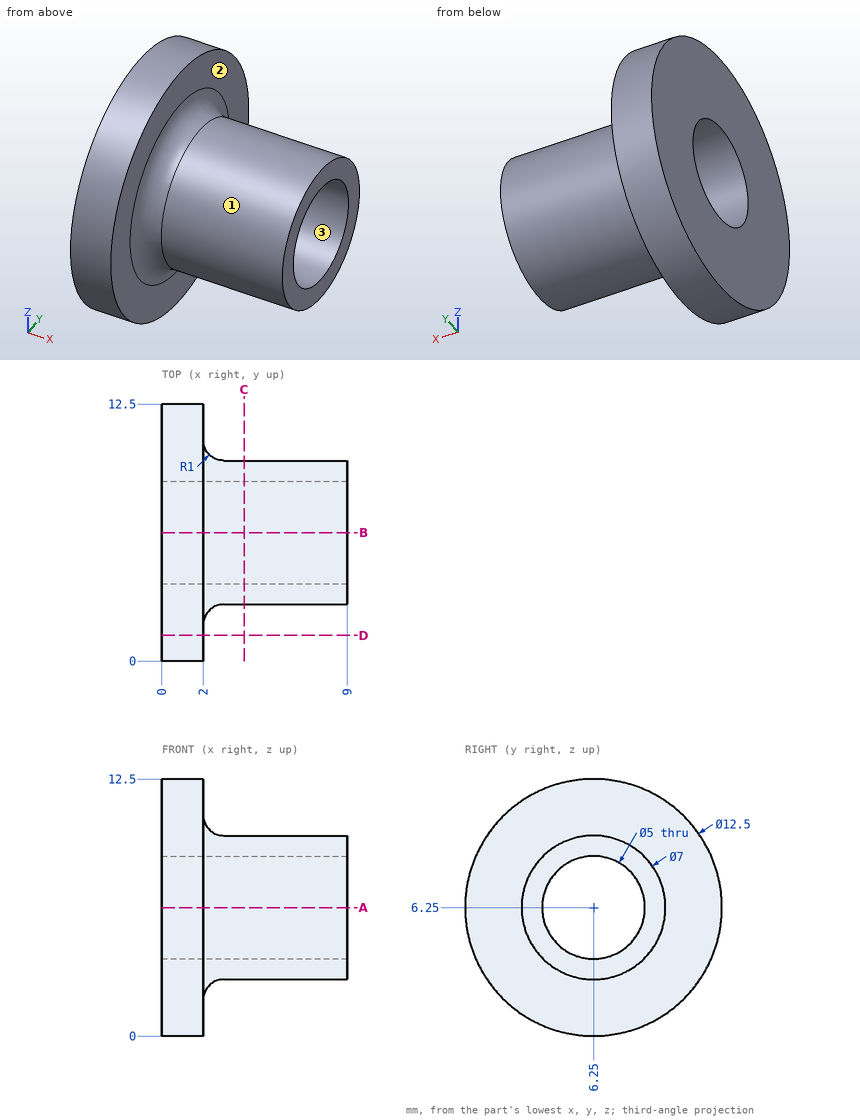
Verification items for this drawing (mm, ordinates from the low corner). Coordinates: 2 decimals unless noted, no trailing zeros. Order: outer loops, then holes, each group sorted by start corner. A loop starts at its lowest first (then second) coordinate and runs counter-clockwise, first axis right, second up. Notation, with made-up numbers: (66.5, 27) - (118.5, 27) arc R33 cw to (118.5, 57) - close; hole circle Ø3 at (44, -24.75). An arc over 180 degrees is marked (long way). Answer as a JSON object with one key per item and string values. Group by question number.
Item 1: Depth check by flat-ended pin: pin 1 Ø5 at (x, y) = (7.5, 9) entering from -Z; pin 2 Ø1 at (y, z) = (7, 4.5) entering from -X; pin 3 Ø2 at (x, y) = (7.5, 6) entering from +Z. Enter the tip coordinate at first touch or a pass-through.
Item 2: Scan lines: probe 1 along Z at (x, y) = (6.5, 6.25); probe 2 along X at (y, z) = (1, 6.5). Record each from-to range of solid material in increasing order.
Item 3: Sectioned sample at A-A, the plane z = 6.25. Record the cut outline in (x, y).
Item 4: Draft check along Y on the marked faces 1, 2 and 3. Enter one of: +Y half, -Y half, draft (parallel to the pull), parting line (faces both ways), or undercut.
Item 5: Sectioned sample at D-D, the plane y = 1.25. Record the cut outline in (x, z).
Item 6: Sectioned sample at C-C, the plane x = 4. Record the cut outline in (y, z), and give its area (3 significant figures).
Resolved:
{
 "1": {"pin 1": "z = 2.76", "pin 2": "through", "pin 3": "z = 9.75"},
 "2": {"probe 1": "2.75 to 3.75, 8.75 to 9.75", "probe 2": "0 to 2"},
 "3": {"outline": "(0, 0) - (2, 0) - (2, 1.75) arc R1 cw to (3, 2.75) - (9, 2.75) - (9, 3.75) - (0, 3.75) - close; (0, 8.75) - (9, 8.75) - (9, 9.75) - (3, 9.75) arc R1 cw to (2, 10.75) - (2, 12.5) - (0, 12.5) - close"},
 "4": {"face 1": "parting line", "face 2": "draft", "face 3": "undercut"},
 "5": {"outline": "(0, 2.5) - (2, 2.5) - (2, 10) - (0, 10) - close"},
 "6": {"outline": "circle Ø7 at (6.25, 6.25); hole circle Ø5 at (6.25, 6.25)", "area": "18.8 mm^2"}
}
